Verification items for the finished model (mm, model axes). A direction names the side the tool comes from. Give positions to 0.01 mm unless a question says otherwise; leave off trailing zeros. Loops run counter-clockwise (first coordinate to the right, second up) from the corner with the lowest first, then second, coordinate; pieces in that order, holes last. Notation, with made-up numbers: (26.5, 1.25) -> (82.5, 1.25) arc R14 ccw to (82.5, 23.25) -> close; hole circle Ø9 at (65, -31). An arc over 180 degrees is marked (long way). Answer in a Markdown table with one row per item. Add a question column.
Q1. Release check for a two-part mould opening along X. For faces 6 (the face through (199, 9, 15)), 7 (the face through (108, 0, 108)), 8 (the face through (219, 9, 108)) record: pulls with the +X half, pulls with the -X half, needs draft (parallel to the pull), parting line crosses it, or undercut.
Q2. Section check B-B on z = 171.5. Enter the section's corners in (x, y).
Q3. Section check D-D on x = 193. Enter the section's corners in (y, z), and give its area (3 significant figures).
Q4. Gauge pin test, flat ends, axial feed: P1, Ø5, axis at x = 79, y = 10, coming from the -Z side; P2, Ø4, axis at x = 109, y = 13, coming from the +Z side; P3, Ø5.5, axis at x = 107, z = 192, coming from the +Y side; P4, Ø9, axis at x = 16.5, y = 13, coming from the +Z side. Record the tip position at first contact, or that the pin passes through.
Q5. Material ranges on probe 1 along X at (y, z) = (12.75, 14); probe 2 along Z at (x, y) = (203, 6); probe 3 along X at (y, z) = (13.5, 205.5), recorded low to high.
Q6. Section check C-C on y = 14. Enter the section's corners in (x, z).
Q7. Set-up check for faces 1 (the face through (109, 12, 144)), 2 (the face through (30, 9, 7)), 3 (the face through (209, 9, 211)), 4 (the face through (214, 9, 219)), 5 (the face through (5, 9, 0)): record each of +Z, -Z, +X, -X, +Y, -Y from which the full face is reachable in a straight line by a thin tool's end or side.
Q8. Section check A-A on x = 110. Enter the section's corners in (y, z), and give its area (3 significant figures).
Autodesk Inventor part; units mm, degrees
ref_plane "YZ Plane" through (0, 0, 0) normal (1, 0, 0) x (0, 1, 0)
ref_plane "XZ Plane" through (0, 0, 0) normal (0, 1, 0) x (-1, 0, 0)
ref_plane "XY Plane" through (0, 0, 0) normal (0, 0, 1) x (1, 0, 0)
sketch "Sketch1" plane through (0, 0, 0) normal (0, 0, 1) x (1, 0, 0)
  line L0 (0, 0) -> (219, 0)
  line L1 (219, 0) -> (219, 18)
  line L2 (219, 18) -> (0, 18)
  line L3 (0, 18) -> (0, 0)
  dimension "d0" = 219
  dimension "d1" = 18
extrude "Extrusion1" add sketch "Sketch1" along normal blind 219
sketch "Sketch2" plane through (0, 0, 219) normal (0, 0, 1) x (1, 0, 0)
  line L0 (102.6988, 18) -> (100.5, 5)
  line L1 (100.5, 5) -> (118.5, 5)
  line L2 (0, 0) -> (219, 0)
  line L3 (219, 18) -> (0, 18)
  line L4 (102.6988, 18) -> (102.6988, 9.1069) construction
  line L5 (109.5, -2.3259) -> (109.5, -4.6671) construction
  line L6 (116.3012, 18) -> (118.5, 5)
  point P0 (109.5, 5)
  point P1 (109.5, 0)
  point P2 (109.5, -3.4965)
  point P3 (109.5, 0)
  dimension "d4" = 5
  dimension "d5" = 9.6
  dimension "d6" = 18
extrude "Extrusion2" cut sketch "Sketch2" against normal blind 75
sketch "Sketch3" plane through (0, 18, 0) normal (0, 1, 0) x (1, 0, 0)
  line L0 (10, -204) -> (30, -204)
  line L1 (0, 0) -> (0, -219)
  line L2 (20, -205.0009) -> (20, -197.8859) construction
  line L3 (102.6988, -219) -> (0, -219) construction
  line L4 (10, -204) -> (10, -219)
  line L5 (30, -204) -> (30, -219)
  line L6 (30, -219) -> (10, -219)
  point P0 (20, -204)
  dimension "d17" = 20
  dimension "d18" = 15
  dimension "d19" = 10
extrude "Extrusion3" cut sketch "Sketch3" against normal through all
pattern_linear "Rectangular Pattern1" count 2 spacing -204 along (0, 0, 1) count 2 spacing 179 along (1, 0, 0) of "Extrusion3"
properties part number "TNS-1-platform"
Taken from the geometry:
| question | item | result |
|---|---|---|
| 1 | face 6 | undercut |
| 1 | face 7 | needs draft |
| 1 | face 8 | pulls with the +X half |
| 2 | outline | (0, 0) -> (219, 0) -> (219, 18) -> (116.3, 18) -> (118.5, 5) -> (100.5, 5) -> (102.7, 18) -> (0, 18) -> close |
| 3 | outline | (0, 15) -> (18, 15) -> (18, 204) -> (0, 204) -> close |
| 3 | area | 3,400 mm² |
| 4 | P1 | stops at z = 0 |
| 4 | P2 | stops at z = 144 |
| 4 | P3 | stops at y = 5 |
| 4 | P4 | stops at z = 204 |
| 5 | probe 1 | x = 0 to 10, 30 to 189, 209 to 219 |
| 5 | probe 2 | z = 15 to 204 |
| 5 | probe 3 | x = 0 to 10, 30 to 101.94, 117.06 to 189, 209 to 219 |
| 6 | outline | (0, 0) -> (10, 0) -> (10, 15) -> (30, 15) -> (30, 0) -> (189, 0) -> (189, 15) -> (209, 15) -> (209, 0) -> (219, 0) -> (219, 219) -> (209, 219) -> (209, 204) -> (189, 204) -> (189, 219) -> (116.98, 219) -> (116.98, 144) -> (102.02, 144) -> (102.02, 219) -> (30, 219) -> (30, 204) -> (10, 204) -> (10, 219) -> (0, 219) -> close |
| 7 | face 1 | +Z |
| 7 | face 2 | -Z, +Y, -Y |
| 7 | face 3 | +Z, +Y, -Y |
| 7 | face 4 | +Z, +X, -X, +Y, -Y |
| 7 | face 5 | -Z, +X, -X, +Y, -Y |
| 8 | outline | (0, 0) -> (18, 0) -> (18, 144) -> (5, 144) -> (5, 219) -> (0, 219) -> close |
| 8 | area | 2,970 mm² |
